Input: part model. Units: mm. Frame: model coordinates. Face numbers are marked on the shaded views. A direction names the side the tool comes from. Coordinates: 2 decimals unless noted, no trailing zeros. Order: outer loops, then holes, each group sorted by start corner. A loop starts at its lowest first (then second) coordinate and runs counter-clockwise, first axis right, second up. Notation, with made-up numbers: (5, 19.25) -> (54, 19.25) arc R11 cw to (54, 36.25) -> close; hole circle Ø3 at (71.25, 40). An arc over 180 degrees is marked (long way). Write each question's results on one line, items separated by ' | '.
```python
from build123d import *

# Parameters (mm, degrees)
SKETCH018_W         = 30.5
SKETCH018_H         = 20
PAD010_DEPTH        = 2.8
PAD011_DEPTH        = 3
PAD012_DEPTH        = 3.5
HOLE005_D           = 4.2
HOLE005_DEPTH       = 25
HOLE005_CSINK_D     = 8.4
HOLE005_CSINK_ANGLE = 90
HOLE005_TIPS_R      = 2.1
POCKET003_DEPTH     = 2.801
CHAMFER001_SIZE     = 2
FILLET001_R         = 0.8


with BuildPart() as part:
    # Sketch018 → Pad010 (new body)
    with BuildSketch(Plane.XY):
        with Locations((18.25, 10)):
            Rectangle(SKETCH018_W, SKETCH018_H)
    extrude(amount=PAD010_DEPTH)

    # Sketch019 (on Face4 of Pad010) → Pad011 (join)
    with BuildSketch(Plane(origin=(3, 0, 0), x_dir=(0, -1, 0), z_dir=(-1, 0, 0))):
        with BuildLine():
            Line((-20, 0), (0, 0))
            Line((0, 0), (0, 12))
            ThreePointArc((0, 12), (-0.585786, 13.414214), (-2, 14))
            Line((-2, 14), (-18, 14))
            ThreePointArc((-18, 14), (-19.414214, 13.414214), (-20, 12))
            Line((-20, 12), (-20, 0))
        make_face()
    extrude(amount=PAD011_DEPTH)

    # Sketch020 (on Face1 of Pad011) → Pad012 (join)
    with BuildSketch(Plane.YZ.offset(33.5)):
        with BuildLine():
            Line((20, 0), (20, 92))
            ThreePointArc((20, 92), (19.414214, 93.414214), (18, 94))
            Line((18, 94), (2, 94))
            ThreePointArc((2, 94), (0.585786, 93.414214), (0, 92))
            Line((0, 92), (0, 0))
            Line((0, 0), (20, 0))
        make_face()
    extrude(amount=PAD012_DEPTH)

    # Hole005
    with Locations(Plane.YZ.offset(37)):
        with Locations((10, 36.5), (10, 86.5)):
            CounterSinkHole(HOLE005_D / 2, HOLE005_CSINK_D / 2, depth=HOLE005_DEPTH, counter_sink_angle=HOLE005_CSINK_ANGLE)

    # Hole005 tips → Hole005 tip 1 section 0
    with BuildSketch(Plane.YZ.offset(12), mode=Mode.PRIVATE) as hole005_tip_1_s0:
        with Locations((10, 36.5)):
            Circle(HOLE005_TIPS_R)
    loft([hole005_tip_1_s0.sketch, Vertex(10.738193, 10, 36.5)], mode=Mode.SUBTRACT)

    # Hole005 tips → Hole005 tip 2 section 0
    with BuildSketch(Plane.YZ.offset(12), mode=Mode.PRIVATE) as hole005_tip_2_s0:
        with Locations((10, 86.5)):
            Circle(HOLE005_TIPS_R)
    loft([hole005_tip_2_s0.sketch, Vertex(10.738193, 10, 86.5)], mode=Mode.SUBTRACT)

    # Sketch022 (on Face1 of Hole005) → Pocket003 (cut, through all)
    with BuildSketch(Plane.XY.offset(2.8)):
        with BuildLine():
            ThreePointArc((16.553834, 12.053193), (14.478422, 9.977781), (16.553834, 7.902369))
            Line((16.553834, 7.902369), (20.553834, 7.902369))
            ThreePointArc((20.553834, 7.902369), (22.629246, 9.977781), (20.553834, 12.053193))
            Line((16.553834, 12.053193), (20.553834, 12.053193))
        make_face()
    extrude(amount=-POCKET003_DEPTH, mode=Mode.SUBTRACT)

    # Chamfer001
    chamfer001_edges = [part.edges().sort_by_distance(p)[0] for p in [
        (18.553834, 7.902369, 2.8),
    ]]
    chamfer(chamfer001_edges, length=CHAMFER001_SIZE)

    # Fillet001
    fillet001_edges = [part.edges().sort_by_distance(p)[0] for p in [
        (0, 10, 14),
        (3, 10, 14),
        (33.5, 10, 94),
        (37, 10, 94),
    ]]
    fillet(fillet001_edges, radius=FILLET001_R)


with BuildPart() as part_1:
    # Body004 placement: moved
    add(part.part.moved(Location((0, -21.9, 0))))


solid = part_1.part
```
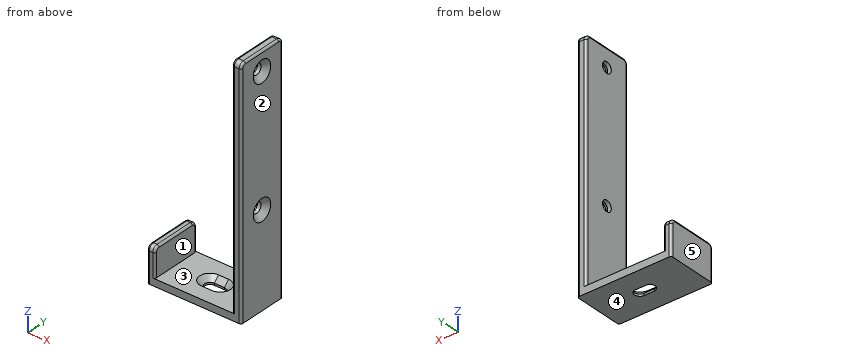
(1) Mould query, pull axis X, two halves, no side actions, for the marked faces 3, 4 and 5. Classes: +X half, -X half, draft (parallel to the pull), parting line (faces both ways), or undercut.
Return value:
face 3: undercut | face 4: draft | face 5: -X half
(2) Cut plane D-D, the plane z = 61. Return loops of the section in (x, y).
Return value:
outline: (33.5, -21.1) arc R0.8 ccw to (34.3, -21.9) -> (36.2, -21.9) arc R0.8 ccw to (37, -21.1) -> (37, -2.7) arc R0.8 ccw to (36.2, -1.9) -> (34.3, -1.9) arc R0.8 ccw to (33.5, -2.7) -> close
(3) Cut plane B-B, the plane y = -5.5. Return loops of the section in (x, z), plus the area to 3 significant figures.
Return value:
outline: (0, 0) -> (37, 0) -> (37, 93.2) arc R0.8 ccw to (36.2, 94) -> (34.3, 94) arc R0.8 ccw to (33.5, 93.2) -> (33.5, 2.8) -> (3, 2.8) -> (3, 13.2) arc R0.8 ccw to (2.2, 14) -> (0.8, 14) arc R0.8 ccw to (0, 13.2) -> close | area: 456 mm2
(4) Cut plane A-A, the plane z = 86.5. Return loops of the section in (x, y).
Return value:
outline: (33.5, -21.1) arc R0.8 ccw to (34.3, -21.9) -> (36.2, -21.9) arc R0.8 ccw to (37, -21.1) -> (37, -16.1) -> (34.9, -14) -> (33.5, -14) -> close; (33.5, -9.8) -> (34.9, -9.8) -> (37, -7.7) -> (37, -2.7) arc R0.8 ccw to (36.2, -1.9) -> (34.3, -1.9) arc R0.8 ccw to (33.5, -2.7) -> close
(5) Reachability of the marked faces 1 and 2 from +Z, -Z, +X, -X, +Y, -Y: full face, straight path, thin tool, end or side. Return the list, or none.
Return value:
face 1: +Z, +Y, -Y | face 2: +Z, -Z, +X, +Y, -Y
(6) Line query: line 1 along Z through (x, y) = (34.65, -11.9); line 2 along Y through (x, z) = (34.3, 86.5); line 3 along X through (y, z) = (-14.25, 10.5). Output: solid intervals per line, ascending. Write a range as from..to.
Return value:
line 1: 0..34.4, 38.6..84.4, 88.6..94 | line 2: -21.9..-14, -9.8..-1.9 | line 3: 0..3, 33.5..37
(7) Pin query (flat end, axial travel): P1, Ø1.5, axis at x = 1.5, y = -11, coming from the +Z side; P2, Ø6, axis at x = 18.5, y = -14, coming from the +Z side; P3, Ø5.5, axis at y = -11.9, z = 86.5, coming from the -X side; P4, Ø5, axis at x = 30.5, z = 31, coming from the -Y side. Return the tip coordinate at first contact, or that it passes through.
Return value:
P1: z = 14 | P2: z = 2.8 | P3: x = 33.5 | P4: through
(8) Cut plane C-C, the plane x = 30.5. Return loops of the section in (y, z), plus the area to 3 significant figures.
Return value:
outline: (-21.9, 0) -> (-1.9, 0) -> (-1.9, 2.8) -> (-21.9, 2.8) -> close | area: 56.0 mm2
